```python
from build123d import *

# Parameters (mm, degrees)
F0_W     = 39.37
F0_H     = 10.16
F1_DEPTH = 7.62
F2_R     = 19.685
F3_DEPTH = 12.7
F4_DEPTH = 3.429
F5_W     = 39.37
F5_H     = 7.62
F6_DEPTH = 3.429


with BuildPart() as f1:
    # F0 (on Top) → F1 (new body)
    with BuildSketch(Plane.XY):
        Rectangle(F0_W, F0_H)
    extrude(amount=F1_DEPTH)

    # F2 (on face) → F3 (cut)
    with BuildSketch(Plane.XZ.offset(5.08)):
        with Locations((0, 22.86)):
            Circle(F2_R)
    extrude(amount=-F3_DEPTH, mode=Mode.SUBTRACT)

    # F2 (on face) → F4 (join)
    with BuildSketch(Plane.XZ.offset(5.08)):
        with BuildLine():
            Line((12.4595997127, 7.62), (-12.4595997127, 7.62))
            ThreePointArc((-12.4595997127, 7.62), (0, 3.175), (12.4595997127, 7.62))
        make_face()
    extrude(amount=-F4_DEPTH)

    # F5 (on face) → F6 (join)
    with BuildSketch(Plane(origin=(0, 5.08, 0), x_dir=(-1, 0, 0), z_dir=(0, 1, 0))):
        with Locations((0, 3.81)):
            Rectangle(F5_W, F5_H)
        with BuildLine():
            Line((-12.4595997127, 7.62), (-19.685, 7.62))
            Line((-19.685, 7.62), (-19.685, 0))
            Line((-19.685, 0), (19.685, 0))
            Line((19.685, 0), (19.685, 7.62))
            Line((19.685, 7.62), (12.4595997127, 7.62))
            ThreePointArc((12.4595997127, 7.62), (0, 3.175), (-12.4595997127, 7.62))
        make_face()
    extrude(amount=-F6_DEPTH)


solid = f1.part
```
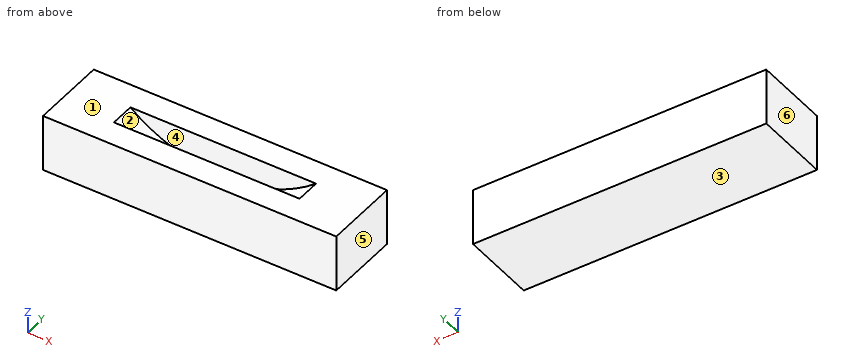
Geometry: final body of the model. Coordinates: model frame, mm. Face numbers are marked on the shaded views. A direction names the side the tool comes from. Coordinates: 2 decimals unless noted, no trailing zeros. Order: outer loops, then holes, each group sorted by start corner. A loop starts at its lowest first (then second) coordinate and runs counter-clockwise, first axis right, second up. Notation, with made-up numbers: (19.25, 18.5) - (33.25, 18.5) arc R21 ccw to (33.25, 53.5) - close; hole circle Ø9 at (4, -19). An arc over 180 degrees is marked (long way). Write each question's results on one line, items separated by ' | '.
1) Pull-direction query (X, two-part tool) for the marked faces 3, 4, 5 and 6; classes: pulls with the +X half, pulls with the -X half, needs draft (parallel to the pull), parting line crosses it, or undercut.
Results list:
face 3: needs draft | face 4: undercut | face 5: pulls with the +X half | face 6: pulls with the -X half
2) Set-up query: the marked faces 1 and 2. Return all of +Z, -Z, +X, -X, +Y, -Y with unobstructed straight access to the full face (end or side cutting, diameter ignored); none if empty.
Results list:
face 1: +Z, +X, -X, +Y, -Y | face 2: +Z
3) Section A-A, the plane z = 6.5. Return loops of the section in (x, y) (3 decimals), plus the area to 3 significant figures.
Results list:
outline: (-19.685, -5.08) - (19.685, -5.08) - (19.685, 5.08) - (-19.685, 5.08) - close; hole (-10.948, -1.651) - (10.948, -1.651) - (10.948, 1.651) - (-10.948, 1.651) - close | area: 328 mm^2
4) Section B-B, the plane x = 6.5. Return loops of the section in (y, z).
Results list:
outline: (-5.08, 0) - (5.08, 0) - (5.08, 7.62) - (1.65, 7.62) - (1.65, 4.28) - (-1.65, 4.28) - (-1.65, 7.62) - (-5.08, 7.62) - close
5) Pin query (flat end, axial travel): pin 1 (5 mm diameter, centred on x = -0.5, y = -1, fed in from +Z). Return the tip coordinate at first contact, or that it passes through.
Results list:
pin 1: z = 7.62
6) Section D-D, the plane z = 4.5. Return loops of the section in (x, y) (3 decimals), plus the area to 3 significant figures.
Results list:
outline: (-19.685, -5.08) - (19.685, -5.08) - (19.685, 5.08) - (-19.685, 5.08) - close; hole (-7.1, -1.651) - (7.1, -1.651) - (7.1, 1.651) - (-7.1, 1.651) - close | area: 353 mm^2
7) Line query: line 1 (Y direction, x = 8.5, z = 5.75); line 2 (X direction, y = -1, z = 6) (3 decimals); line 3 (Z direction, x = 4.5, y = -1). Output: solid intervals per line, ascending. Write a range as from..to.
Results list:
line 1: -5.08..-1.65, 1.65..5.08 | line 2: -19.685..-10.161, 10.161..19.685 | line 3: 0..3.7
8) Section C-C, the plane y = -0.5. Return loops of the section in (x, z) (3 decimals).
Results list:
outline: (-19.685, 0) - (19.685, 0) - (19.685, 7.62) - (12.46, 7.62) arc R19.685 cw to (-12.46, 7.62) - (-19.685, 7.62) - close
